Autodesk Inventor part; units mm, degrees
ref_plane "YZ Plane" through (0, 0, 0) normal (1, 0, 0) x (0, 1, 0)
ref_plane "XZ Plane" through (0, 0, 0) normal (0, 1, 0) x (-1, 0, 0)
ref_plane "XY Plane" through (0, 0, 0) normal (0, 0, 1) x (1, 0, 0)
sketch "Esquisse1" plane through (0, 0, 0) normal (0, 1, 0) x (-1, 0, 0)
  line L0 (7.2872, 10.2128) -> (-22.7128, 10.2128)
  line L1 (-22.7128, 10.2128) -> (-22.7128, -19.7872)
  line L2 (-22.7128, -19.7872) -> (7.2872, -19.7872)
  line L3 (7.2872, -19.7872) -> (7.2872, 10.2128)
  point P0 (0, 0)
  dimension "d0" = 30
  dimension "d1" = 30
extrude "Extrusion1" add sketch "Esquisse1" along normal blind 23
ref_plane "Plan médian" through (7.7128, 0, 10.2128) normal (1, 0, 0) x (0, 0, -1)
sketch "Esquisse4" plane through (0, 0, 0) normal (0, -1, 0) x (1, 0, 0)
  circle A0 centre (7.7128, -7.8122) radius 11.975
  line L0 (-7.2872, 10.2128) -> (22.7128, 10.2128)
  line L1 (4.1002, 3.6049) -> (4.1002, 10.2128)
  line L2 (11.3254, 3.6049) -> (11.3254, 10.2128)
  point P0 (0, 0)
extrude "Extrusion2" cut sketch "Esquisse4" against normal blind 22
sketch "Esquisse5" plane through (0, 22, 0) normal (0, -1, 0) x (1, 0, 0)
  circle A0 centre (15.507, -3.3122) radius 1.25
  circle A1 centre (-0.0815, -3.3122) radius 1.25
  circle A2 centre (7.7128, -16.8122) radius 1.25
  circle A3 centre (7.7128, -7.8122) radius 6
  point P0 (0, 0)
extrude "Extrusion3" cut sketch "Esquisse5" against normal through all
sketch "Esquisse6" plane through (-7.2872, 23, 10.2128) normal (0, 0, 1) x (1, 0, 0)
  line L0 (0, -23) -> (11.3874, -23)
  line L1 (5.9558, 0) -> (8.4558, 0)
  line L2 (0, -23) -> (7, -23)
  line L3 (7, -23) -> (7, 0)
  line L4 (7, 0) -> (0, 0)
  line L5 (0, 0) -> (0, -23)
  line L6 (30, -23) -> (30, 0)
  line L7 (0, 0) -> (30, 0)
  line L8 (30, -23) -> (23, -23)
  line L9 (23, -23) -> (23, 0)
  line L10 (23, 0) -> (30, 0)
  line L11 (30, 0) -> (30, -23)
  point P0 (7.2872, -23)
  point P1 (12, -23)
  point P2 (11.5355, -23)
  dimension "d8" = 7
  dimension "d9" = 7
extrude "Extrusion4" add sketch "Esquisse6" along normal blind 10
sketch "Esquisse7" plane through (-7.2872, 23, 20.2128) normal (0, 0, 1) x (1, 0, 0)
  line L0 (7, 0) -> (-20, 0)
  line L1 (-20, 0) -> (-20, -23)
  line L2 (-20, -23) -> (7, -23)
  line L3 (7, -23) -> (7, 0)
  line L4 (30, 0) -> (0, 0)
  line L5 (23, 0) -> (50, 0)
  line L6 (50, 0) -> (50, -23)
  line L7 (50, -23) -> (23, -23)
  line L8 (23, -23) -> (23, 0)
  line L9 (0, 0) -> (0, -23)
  line L10 (30, -23) -> (30, 0)
  point P0 (7.2872, -23)
  dimension "d12" = 20
  dimension "d13" = 20
extrude "Extrusion5" add sketch "Esquisse7" along normal blind 5
sketch "Esquisse8" plane through (0, 23, 0) normal (0, 1, 0) x (1, 0, 0)
  line L0 (36.2128, -25.2128) -> (31.2128, -25.2128)
  line L1 (31.2128, -25.2128) -> (31.2128, -20.2128)
  line L2 (31.2128, -20.2128) -> (36.2128, -20.2128)
  line L3 (36.2128, -20.2128) -> (36.2128, -25.2128)
  line L4 (42.7128, -20.2128) -> (42.7128, -25.2128)
  line L5 (42.7128, -20.2128) -> (22.7128, -20.2128)
  line L6 (-0.2872, -25.2128) -> (-27.2872, -25.2128)
  line L7 (-27.2872, -20.2128) -> (-27.2872, -25.2128)
  line L8 (-20.7872, -25.2128) -> (-15.7872, -25.2128)
  line L9 (-15.7872, -25.2128) -> (-15.7872, -20.2128)
  line L10 (-15.7872, -20.2128) -> (-20.7872, -20.2128)
  line L11 (-20.7872, -20.2128) -> (-20.7872, -25.2128)
  line L12 (-7.2872, -20.2128) -> (-27.2872, -20.2128)
  point P0 (0, 0)
  point P1 (-0.4939, -25.2128)
  dimension "d16" = 6.5
  dimension "d17" = 5
  dimension "d18" = 5
  dimension "d19" = 0
  dimension "d53" = 5
  dimension "d54" = 5
  dimension "d55" = 0
  dimension "d57" = 6.5
extrude "Extrusion6" add sketch "Esquisse8" along normal blind 3 contours L0 L1 L2 L3 | L6 L11 L10 L9
sketch "Esquisse9" plane through (0, 26, 0) normal (0, 1, 0) x (1, 0, 0)
  line L0 (37.7128, -26.7128) -> (29.7128, -26.7128)
  line L1 (29.7128, -26.7128) -> (29.7128, -18.7128)
  line L2 (29.7128, -18.7128) -> (37.7128, -18.7128)
  line L3 (37.7128, -18.7128) -> (37.7128, -26.7128)
  line L4 (42.7128, -20.2128) -> (42.7128, -25.2128)
  line L5 (-27.2872, -25.2128) -> (-0.2872, -25.2128)
  line L6 (-27.2872, -20.2128) -> (-27.2872, -25.2128)
  line L7 (31.2128, -25.2128) -> (15.7128, -25.2128)
  line L8 (-14.2872, -26.7128) -> (-22.2872, -26.7128)
  line L9 (-22.2872, -26.7128) -> (-22.2872, -18.7128)
  line L10 (-22.2872, -18.7128) -> (-14.2872, -18.7128)
  line L11 (-14.2872, -18.7128) -> (-14.2872, -26.7128)
  point P0 (0, 0)
  point P1 (-13.7872, -25.2128)
  dimension "d25" = 8
  dimension "d26" = 5
  dimension "d59" = 8
  dimension "d60" = 1.5
  dimension "d62" = 5
  dimension "d63" = 1.5
  dimension "d64" = 8
  dimension "d65" = 8
extrude "Extrusion7" add sketch "Esquisse9" along normal blind 3
sketch "Esquisse10" plane through (22.7128, 23, -19.7872) normal (0, 0, -1) x (-1, 0, 0)
  line L0 (0, -23) -> (15, -23)
  line L1 (15, -23) -> (15, -1)
  line L2 (15, -23) -> (30, -23)
  line L3 (30, -23) -> (30, 0)
  line L4 (0, 0) -> (30, 0)
  line L5 (0, -23) -> (0, 0)
  line L6 (0, 0) -> (30, 0)
  line L7 (30, 0) -> (30, -23)
  line L8 (30, -23) -> (0, -23)
  line L9 (0, -23) -> (0, 0)
  point P0 (22.7128, -23)
extrude "Extrusion8" add sketch "Esquisse10" along normal blind 2
fillet "Congé1" radius 10 2 edges at (22.7128, 11.5, -21.7872) (-7.2872, 11.5, -21.7872)
sketch "Esquisse12" plane through (0, 0, 0) normal (0, -1, 0) x (1, 0, 0)
  arc A0 (4.1002, 3.6049) -> (11.3254, 3.6049) centre (7.7128, -7.8122) ccw
  circle A1 centre (7.7128, -7.8122) radius 12.5
  point P0 (0, 0)
  dimension "d42" = 25
extrude "Extrusion10" cut sketch "Esquisse12" against normal up to surface (22 mm away)
sketch "Esquisse13" plane through (-7.2872, 23, 25.2128) normal (0, 0, 1) x (1, 0, 0)
  circle A0 centre (-11, -8) radius 1.5
  circle A1 centre (41, -8) radius 1.5
  line L0 (7, 0) -> (-20, 0)
  line L1 (-20, 0) -> (-20, -23)
  line L2 (50, 0) -> (23, 0)
  line L3 (50, -23) -> (50, 0)
  point P0 (7.2872, -23)
  dimension "d45" = 3
  dimension "d46" = 3
  dimension "d49" = 8
  dimension "d50" = 9
  dimension "d51" = 8
  dimension "d52" = 9
extrude "Extrusion11" cut sketch "Esquisse13" against normal through all
sketch "Esquisse14" plane through (0, 0, 0) normal (0, -1, 0) x (1, 0, 0)
  line L0 (15.7128, 25.2128) -> (42.7128, 25.2128)
  line L1 (22.7128, 20.2128) -> (42.7128, 20.2128)
  line L2 (-20.7872, 25.2128) -> (-15.7872, 25.2128)
  line L3 (-15.7872, 25.2128) -> (-15.7872, 20.2128)
  line L4 (-15.7872, 20.2128) -> (-20.7872, 20.2128)
  line L5 (-20.7872, 20.2128) -> (-20.7872, 25.2128)
  line L6 (-27.2872, 20.2128) -> (-27.2872, 25.2128)
  line L7 (31.2128, 25.2128) -> (36.2128, 25.2128)
  line L8 (36.2128, 25.2128) -> (36.2128, 20.2128)
  line L9 (36.2128, 20.2128) -> (31.2128, 20.2128)
  line L10 (31.2128, 20.2128) -> (31.2128, 25.2128)
  line L11 (42.7128, 20.2128) -> (42.7128, 25.2128)
  point P0 (0, 0)
  dimension "d66" = 6.5
  dimension "d67" = 5
  dimension "d69" = 5
  dimension "d70" = 6.5
  dimension "d71" = 5
  dimension "d72" = 5
  dimension "d73" = 0
extrude "Extrusion12" add sketch "Esquisse14" along normal blind 3 contours L0 L8 L1 L10 | L2 L3 L4 L5
sketch "Esquisse15" plane through (0, -3, 0) normal (0, -1, 0) x (1, 0, 0)
  line L0 (-22.2872, 26.7128) -> (-14.2872, 26.7128)
  line L1 (-14.2872, 26.7128) -> (-14.2872, 18.7128)
  line L2 (-14.2872, 18.7128) -> (-22.2872, 18.7128)
  line L3 (-22.2872, 18.7128) -> (-22.2872, 26.7128)
  line L4 (29.7128, 26.7128) -> (37.7128, 26.7128)
  line L5 (37.7128, 26.7128) -> (37.7128, 18.7128)
  line L6 (37.7128, 18.7128) -> (29.7128, 18.7128)
  line L7 (29.7128, 18.7128) -> (29.7128, 26.7128)
  line L8 (-27.2872, 20.2128) -> (-27.2872, 25.2128)
  line L9 (-27.2872, 20.2128) -> (-20.7872, 20.2128)
  line L10 (42.7128, 20.2128) -> (42.7128, 25.2128)
  line L11 (36.2128, 20.2128) -> (42.7128, 20.2128)
  point P0 (0, 0)
  dimension "d76" = 8
  dimension "d77" = 8
  dimension "d78" = 8
  dimension "d79" = 8
  dimension "d80" = 5
  dimension "d81" = 1.5
  dimension "d82" = 5
  dimension "d83" = 1.5
extrude "Extrusion13" add sketch "Esquisse15" along normal blind 3
properties part number "support_codeur"
The listing builds one solid part. Answer for the finished solid, in the listing's coordinates (mm). A direction names the side the tool comes from. Give positions to 0.01 mm unless a question says otherwise; leave off trailing zeros. Write each loop counter-clockwise with the first axis right and the second up, starting at its lowest first coordinate (ties: lowest second). Pieces come first, ordered by that corner, then holes. Notation, with made-up numbers: (-37, -25.5) - (-11, -25.5) arc R34 ccw to (-11, 8.5) - close; hole circle Ø8 at (17, -28). An arc over 180 degrees is marked (long way). One line per question, with ' | ' between items. Start each with the question number.
1. Section A-A, the plane z = 11.5 is taken. Determine the outline of the cut face in (x, y), then the cut area to 3 significant figures.
2. Straight lines are drawn through the part: line 1 (X direction, y = 12, z = 17.5); line 2 (X direction, y = 3, z = 8); line 3 (Z direction, x = -11.5, y = 16). For each, find the intervals that lie inside material, in ascending order.
3. Section D-D, the plane y = 1.5 is taken. Determine the outline of the cut face in (x, z).
4. For faces 4 (the face through (-22.287, 27, 23)), 5 (the face through (29.713, 27, 23)), 6 (the face through (40, 0, 23)), 7 (the face through (34, 26, 20)), 8 (the face through (-24, 0, 23)), determine the directions among +Z, -Z, +X, -X, +Y, -Y from which every point of the face is accessible in a straight line to the end or side of a thin tool.
5. Section B-B, the plane y = 15 is taken. Determine the outline of the cut face in (x, z).
6. Given P1, Ø0.9, axis at y = 24.5, z = 23, coming from the -X side; P2, Ø5, axis at x = -10, y = 8, coming from the +Z side; P3, Ø7, axis at x = 7.71, z = -7.81, coming from the -Y side; P4, Ø2.5, axis at y = -4.5, z = 23.5, coming from the -X side, each flat-ended and moving along its own axis, determine where each tip first touches the part or whether it passes through.
7. Section C-C, the plane x = -19 is taken. Determine the outline of the cut face in (y, z).
8. Determine the mould class of faces 1 (the face through (-18, -4, 18.713)), 2 (the face through (40, 23, 23)), 3 (the face through (-0.244, 22.493, -2.073)) for opening direction Z: +Z half, -Z half, draft (parallel to the pull), parting line (faces both ways), or undercut.
Result:
1) outline: (-7.29, 0) - (-0.29, 0) - (-0.29, 23) - (-7.29, 23) - close; (15.71, 0) - (22.71, 0) - (22.71, 23) - (15.71, 23) - close | area: 322 mm2
2) line 1: x = -7.29 to -0.29, 15.71 to 22.71 | line 2: x = -7.29 to 4.1, 11.33 to 22.71 | line 3: z = 20.21 to 25.21
3) outline: (-27.29, 20.21) - (-7.29, 20.21) - (-7.29, -11.79) arc R10 ccw to (2.71, -21.79) - (12.71, -21.79) arc R10 ccw to (22.71, -11.79) - (22.71, 20.21) - (42.71, 20.21) - (42.71, 25.21) - (15.71, 25.21) - (15.71, 10.21) - (11.33, 10.21) - (11.33, 4.15) arc R12.5 cw (long way) to (4.1, 4.15) - (4.1, 10.21) - (-0.29, 10.21) - (-0.29, 25.21) - (-27.29, 25.21) - close
4) face 4: +Z, -Z, -X, +Y | face 5: +Z, -Z, +Y | face 6: +Z, -Z, +X | face 7: none | face 8: +Z, -Z, -X
5) outline: (-27.29, 20.21) - (-19.79, 20.21) - (-19.79, 25.21) - (-27.29, 25.21) - close; (-16.79, 20.21) - (-7.29, 20.21) - (-7.29, -11.79) arc R10 ccw to (2.71, -21.79) - (12.71, -21.79) arc R10 ccw to (22.71, -11.79) - (22.71, 20.21) - (32.21, 20.21) - (32.21, 25.21) - (15.71, 25.21) - (15.71, 10.21) - (11.33, 10.21) - (11.33, 4.15) arc R12.5 cw (long way) to (4.1, 4.15) - (4.1, 10.21) - (-0.29, 10.21) - (-0.29, 25.21) - (-16.79, 25.21) - close; (35.21, 20.21) - (42.71, 20.21) - (42.71, 25.21) - (35.21, 25.21) - close
6) P1: stops at x = -20.79 | P2: stops at z = 25.21 | P3: passes through | P4: stops at x = -22.29
7) outline: (-6, 18.71) - (-3, 18.71) - (-3, 20.21) - (13.68, 20.21) - (13.68, 25.21) - (-3, 25.21) - (-3, 26.71) - (-6, 26.71) - close; (16.32, 20.21) - (26, 20.21) - (26, 18.71) - (29, 18.71) - (29, 26.71) - (26, 26.71) - (26, 25.21) - (16.32, 25.21) - close
8) face 1: -Z half | face 2: draft | face 3: undercut
